Check sheet for the modelled part. Datum: model origin and axes. Units: mm. Face numbers are marked on the shaded views. A direction names the side the tool comes from. Round coordinates to 2 decimals unless told otherwise and drop trailing zeros. Write each loop counter-clockwise with the first axis right and the second up, starting at its lowest first coordinate (ties: lowest second). Pieces come first, ordered by that corner, then holes.
Item 1: Release check for a two-part mould opening along Z. For the marked faces 1, 2 and 3 record: pulls with the +Z half, pulls with the -Z half, needs draft (parallel to the pull), parting line crosses it, or undercut.
Item 2: Section check C-C, the plane z = 0. Record the cut outline in (x, y).
Item 3: Depth check by flat-ended pin: pin 1 (1.5 mm diameter, centred on y = -1.5, z = -2, fed in from -X); pin 2 (1.5 mm diameter, centred on x = 13, z = 0, fed in from +Y); pin 3 (1 mm diameter, centred on y = 1.5, z = 2.5, fed in from +X); pin 4 (3 mm diameter, centred on y = -1.5, z = -2, fed in from -X). Enter the tip coordinate at first touch or a pass-through.
Item 4: Material ranges on line 1 along Y through (x, z) = (5.75, 0.9); line 2 along X through (y, z) = (1.25, -0.1); line 3 along X through (y, z) = (2, 0.55), recorded low to high.
Item 5: Section check B-B, the plane y = -2. Record the cut outline in (x, z).
Item 6: Set-up check for the marked faces 4, 5, 6, 7 and 8: record each of +Z, -Z, +X, -X, +Y, -Y from which the full face is reachable in a straight line by a thin tool's end or side.
Item 7: Section check A-A, the plane x = 15. Record the cut outline in (y, z), plus the area to 3 significant figures.
Item 8: Section check D-D, the plane x = 0. Record the cut outline in (y, z), plus the area to 3 significant figures.
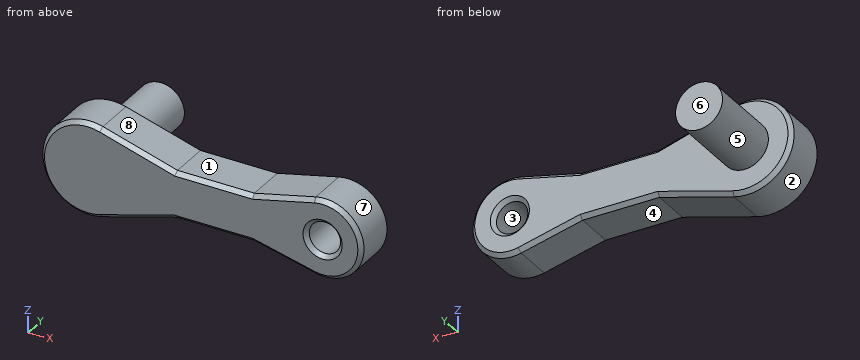
from build123d import *

# Parameters (mm, degrees)
SKETCH_1_R          = 1.5
EXTRUDE_1_DEPTH     = 5
EXTRUDE_3_DEPTH     = 3
SKETCH_5_R          = 1
CUT_EXTRUDE_2_DEPTH = 3
EXTRUDE_4_DEPTH     = 3
EXTRUDE_5_DEPTH     = 3
CHAMFER_2_SIZE      = 0.25


with BuildPart() as part:
    # 草图1 → 凸台-拉伸1 (new body)
    with BuildSketch(Plane(origin=(0, 0, 0), x_dir=(1, 0, 0), z_dir=(0, 1, 0))):
        with Locations(Location((0, 0, 0), (0, 0, 270))):
            Circle(SKETCH_1_R)
    extrude(amount=EXTRUDE_1_DEPTH)

    # 草图4 → 凸台-拉伸3 (add)
    with BuildSketch(Plane(origin=(0, 0, 0), x_dir=(1, 0, 0), z_dir=(0, 1, 0))):
        with BuildLine():
            Line((2.598076211, 1.5), (13, 1.5))
            ThreePointArc((13, 1.5), (17.5, 0), (13, -1.5))
            Line((13, -1.5), (2.598076211, -1.5))
            ThreePointArc((2.598076211, -1.5), (-3, 0), (2.598076211, 1.5))
        make_face()
    extrude(amount=-EXTRUDE_3_DEPTH)

    # 草图5 → 切除-拉伸2 (cut)
    with BuildSketch(Plane(origin=(0, 0, 0), x_dir=(1, 0, 0), z_dir=(0, 1, 0))):
        with Locations(Location((15, 0, 0), (0, 0, 270))):
            Circle(SKETCH_5_R)
    extrude(amount=-CUT_EXTRUDE_2_DEPTH, mode=Mode.SUBTRACT)

    # 草图7 → 凸台-拉伸4 (add)
    with BuildSketch(Plane(origin=(0, 0, 0), x_dir=(1, 0, 0), z_dir=(0, 1, 0))):
        with BuildLine():
            Line((10.5, 1.5), (14.421854812, 2.432231104))
            ThreePointArc((14.421854812, 2.432231104), (13.629244055, 2.090700395), (13, 1.5))
            Line((13, 1.5), (10.5, 1.5))
        make_face()
        with BuildLine():
            Line((10.5, -1.5), (14.421854812, -2.432231104))
            ThreePointArc((14.421854812, -2.432231104), (13.629244055, -2.090700395), (13, -1.5))
            Line((13, -1.5), (10.5, -1.5))
        make_face()
    extrude(amount=-EXTRUDE_4_DEPTH)

    # 草图9 → 凸台-拉伸5 (add)
    with BuildSketch(Plane(origin=(0, 0, 0), x_dir=(1, 0, 0), z_dir=(0, 1, 0))):
        with BuildLine():
            Line((5.598076211, 1.5), (2.598076211, 1.5))
            ThreePointArc((2.598076211, 1.5), (1.850570943, 2.36122578), (0.835663526, 2.881261264))
            Line((0.835663526, 2.881261264), (5.598076211, 1.5))
        make_face()
        with BuildLine():
            Line((2.598076211, -1.5), (5.598076211, -1.5))
            Line((5.598076211, -1.5), (0.835663526, -2.881261264))
            ThreePointArc((0.835663526, -2.881261264), (1.850570943, -2.36122578), (2.598076211, -1.5))
        make_face()
    extrude(amount=-EXTRUDE_5_DEPTH)

    # 倒角2
    chamfer_2_edges = [part.edges().sort_by_distance(p)[0] for p in [
        (15, 0, -1),
        (15, -3, -1),
        (17.5, 0, 0),
        (17.5, -3, 0),
        (12.460927406, 0, 1.966115552),
        (12.460927406, -3, 1.966115552),
        (8.049038106, 0, -1.5),
        (8.049038106, -3, -1.5),
        (12.460927406, 0, -1.966115552),
        (12.460927406, -3, -1.966115552),
        (-3, 0, 0),
        (-3, -3, 0),
        (3.216869869, 0, -2.190630632),
        (3.216869869, -3, -2.190630632),
        (8.049038106, 0, 1.5),
        (8.049038106, -3, 1.5),
        (3.216869869, 0, 2.190630632),
        (3.216869869, -3, 2.190630632),
    ]]
    chamfer(chamfer_2_edges, length=CHAMFER_2_SIZE)


solid = part.part
Values found:
1. face 1: pulls with the +Z half
1. face 2: parting line crosses it
1. face 3: undercut
2. outline: (-3, -2.75) - (-2.75, -3) - (13.75, -3) - (14, -2.75) - (14, -0.25) - (13.75, 0) - (1.5, 0) - (1.5, 5) - (-1.5, 5) - (-1.5, 0) - (-2.75, 0) - (-3, -0.25) - close; (16, -2.75) - (16.25, -3) - (17.25, -3) - (17.5, -2.75) - (17.5, -0.25) - (17.25, 0) - (16.25, 0) - (16, -0.25) - close
3. pin 1: stops at x = -2.73
3. pin 2: stops at y = 0
3. pin 3: passes through
3. pin 4: stops at x = -2.96
4. line 1: y = -3 to 0
4. line 2: x = -1.5 to 1.5
4. line 3: x = -1.4 to 1.4
5. outline: (0.84, -2.88) - (5.6, -1.5) - (10.5, -1.5) - (14.42, -2.43) arc R2.5 ccw (long way) to (14.42, 2.43) - (10.5, 1.5) - (5.6, 1.5) - (0.84, 2.88) arc R3 ccw (long way) to start; hole circle Ø2 at (15, 0)
6. face 4: -Z, +Y, -Y
6. face 5: +Y
6. face 6: +Z, -Z, +X, -X, +Y
6. face 7: +Y, -Y
6. face 8: +Z, +Y, -Y
7. outline: (-3, -2.25) - (-2.75, -2.5) - (-0.25, -2.5) - (0, -2.25) - (0, -1.25) - (-0.25, -1) - (-2.75, -1) - (-3, -1.25) - close; (-3, 1.25) - (-2.75, 1) - (-0.25, 1) - (0, 1.25) - (0, 2.25) - (-0.25, 2.5) - (-2.75, 2.5) - (-3, 2.25) - close
7. area: 8.75 mm2
8. outline: (-3, -2.75) - (-2.75, -3) - (-0.25, -3) - (0, -2.75) - (0, -1.5) - (5, -1.5) - (5, 1.5) - (0, 1.5) - (0, 2.75) - (-0.25, 3) - (-2.75, 3) - (-3, 2.75) - close
8. area: 32.9 mm2
